from build123d import *

# Parameters (mm, degrees)
F2_R     = 4
F3_DEPTH = 25
F5_SIZE  = 1
F6_R     = 1


# Not quite as in the source:
# - a fillet or chamfer that OpenCascade refuses, or shapes differently, is made with other operations: its cross-section is extruded or revolved along the edge and cut away or added


with BuildPart() as f1:
    # F0 (on Front) → F1 (revolve)
    with BuildSketch(Plane.XZ):
        Polygon((-10, 0), (0, 0), (0, 3), (-10, 3), (-10, 6), (-15, 6), (-15, -7), (-10, -7), align=None)
    revolve(axis=Axis((0, 0, 1.5), (0, 0, -1)))

    # F2 (on face) → F3 (cut)
    with BuildSketch(Plane.XY.offset(3)):
        Circle(F2_R)
    extrude(amount=-F3_DEPTH, mode=Mode.SUBTRACT)

    # F4: fillet of radius 2 on 1 edges, made by hand

    # F4_s1 → F4_t2 (revolve, cut)
    with BuildSketch(Plane.XZ):
        with BuildLine():
            add(Edge.make_bspline(
                [(-10, 4), (-10, 6), (-12, 6)],
                knots=[0, 0, 0, 1, 1, 1], degree=2, weights=[1, 0.25, 1]))
            Line((-12, 6), (-10, 6))
            Line((-10, 6), (-10, 4))
        make_face()
    revolve(axis=Axis((0, 0, 6), (0, 0, -1)), mode=Mode.SUBTRACT)

    # F5
    f5_edges = [f1.edges().sort_by_distance(p)[0] for p in [
        (15, 0, 6),
    ]]
    chamfer(f5_edges, length=F5_SIZE)

    # F6
    f6_edges = [f1.edges().sort_by_distance(p)[0] for p in [
        (14, 0, 6),
    ]]
    fillet(f6_edges, radius=F6_R)

    # F7: fillet of radius 1 on 1 edges, made by hand

    # F7_s1 → F7_t2 (revolve, cut)
    with BuildSketch(Plane.XZ):
        with BuildLine():
            add(Edge.make_bspline(
                [(-14.7071067812, 5.2928932188), (-15, 5), (-15, 4.5857864376)],
                knots=[0, 0, 0, 1, 1, 1], degree=2, weights=[1, 1, 1]))
            Line((-15, 4.5857864376), (-15, 5))
            Line((-15, 5), (-14.7071067812, 5.2928932188))
        make_face()
    revolve(axis=Axis((0, 0, 5), (0, 0, -1)), mode=Mode.SUBTRACT)


solid = f1.part
Source: CAD feature listing. Evaluate the final solid. Frame: model axes, mm. A direction names the side the tool comes from. Round coordinates to 2 decimals unless told otherwise and drop trailing zeros. Loops run counter-clockwise (first coordinate to the right, second up) from the corner with the lowest first, then second, coordinate; pieces in that order, holes last.
Q1. Ray query, line 1 (Y direction, x = 0, z = 1.65); line 2 (Y direction, x = 0, z = -2.5); line 3 (Z direction, x = -9, y = -2). Return the intervals inside material, ascending.
Q2. Section B-B, the plane z = -5. Return loops of the section in (x, y), plus the area to 3 significant figures.
Q3. First-contact query: P1, Ø6, axis at y = 11.5, z = 1.5, coming from the +X side; P2, Ø16, axis at x = -0.5, y = -3, coming from the +Z side; P3, Ø1.5, axis at x = -11.5, z = 1.5, coming from the -Y side. Flat tips, straight axial feed; report the tip coordinate or a pass-through.
Q4. Section A-A, the plane z = 2. Return loops of the section in (x, y), plus the area to 3 significant figures.
Q5. Mould query, pull axis X, two halves, no side actions, for faces 4 (the face through (14.985, 0.66, -1.288)), 5 (the face through (7, -10, 6)), 6 (the face through (4.3, 0.1, 3)). Classes: pulls with the +X half, pulls with the -X half, needs draft (parallel to the pull), parting line crosses it, or undercut.
Q6. Access query for faces 1 (the face through (2.17, -9.76, -3.45)), 2 (the face through (-3, -10, -7)), 3 (the face through (2.17, -9.76, 3.51)). Directions: +Z, -Z, +X, -X, +Y, -Y. A direction counts if a zero-diameter tool reaches every point of the face in a straight line with its end or side. Return the directions, or none.
Solutions:
1. line 1: y = -15 to -4, 4 to 15
1. line 2: y = -15 to -10, 10 to 15
1. line 3: z = 0 to 3
2. outline: circle Ø30 at (0, 0); hole circle Ø20 at (0, 0)
2. area: 393 mm2
3. P1: stops at x = 12.36
3. P2: stops at z = 5.43
3. P3: stops at y = -10.46
4. outline: circle Ø30 at (0, 0); hole circle Ø8 at (0, 0)
4. area: 657 mm2
5. face 4: parting line crosses it
5. face 5: needs draft
5. face 6: undercut
6. face 1: -Z
6. face 2: -Z, +X, -X, +Y, -Y
6. face 3: +Z
